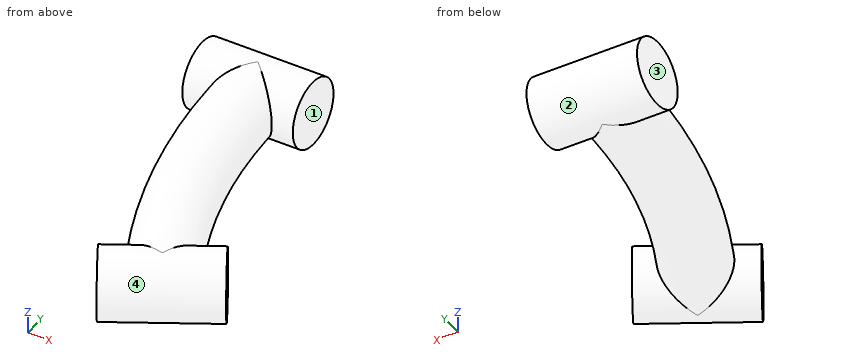
```python
from build123d import *

# Parameters (mm, degrees)
F0_R     = 3.81
F4_R     = 3.81
F5_DEPTH = 6.35
F8_R     = 3.81
F9_DEPTH = 6.35


with BuildPart() as f2:
    # F2: sweep along a path in F1
    with BuildLine(Plane.XY) as f2_path:
        ThreePointArc((0, 0), (2.5964520368, -19.7220112368), (10.2088642316, -38.1))
    # F0 (on Front) → F2 (sweep)
    with BuildSketch(Plane.XZ):
        with Locations((12.7, 0)):
            Circle(F0_R)
    sweep(path=f2_path.line)

    # F4 (on offset) → F5 (join, symmetric)
    with BuildSketch(Plane.YZ.offset(12.7)):
        Circle(F4_R)
    extrude(amount=F5_DEPTH, both=True)

    # F8 (on face) → F9 (join, symmetric)
    with BuildSketch(Plane(origin=(2.1573868597, 1.2455678842, 0), x_dir=(-0.5, 0.8660254038, 0), z_dir=(0.8660254038, 0.5, 0))):
        with Locations((-38.1, 0)):
            Circle(F8_R)
    extrude(amount=F9_DEPTH, both=True)


solid = f2.part
```
Work out the finished part from the listing and answer in its coordinate system (mm). Face numbers are marked on the shaded views. A direction names the side the tool comes from. Give positions to 0.01 mm unless a question says otherwise; leave off trailing zeros. Order: outer loops, then holes, each group sorted by start corner. A loop starts at its lowest first (then second) coordinate and runs counter-clockwise, first axis right, second up.
1. Section B-B, the plane z = -2.25 is taken. Determine the outline of the cut face in (x, y), and give its area (3 significant figures).
Result sheet:
outline: (6.35, -3.07) - (9.7, -3.07) arc R66.57 ccw to (17.07, -30.59) - (14.17, -32.26) - (17.25, -37.59) - (28.24, -31.24) - (25.17, -25.91) - (22.4, -27.51) arc R60.43 cw to (15.85, -3.07) - (19.05, -3.07) - (19.05, 3.07) - (6.35, 3.07) - close
area: 323 mm2
2. For the marked faces 1 and 2, determine the directions among +Z, -Z, +X, -X, +Y, -Y from which every point of the face is accessible in a straight line to the end or side of a thin tool.
Result sheet:
face 1: +Z, -Z, +X, +Y
face 2: none
3. Section A-A, the plane z = 1.5 is taken. Determine the outline of the cut face in (x, y).
Result sheet:
outline: (6.35, -3.5) - (9.29, -3.5) arc R67 ccw to (16.5, -30.42) - (13.96, -31.89) - (17.46, -37.96) - (28.46, -31.61) - (24.96, -25.54) - (22.58, -26.91) arc R60 cw to (16.3, -3.5) - (19.05, -3.5) - (19.05, 3.5) - (6.35, 3.5) - close
4. The mould has two halves that part along Y. Classify the marked faces 3 and 4: released by +Y, released by -Y, zero draft, split by the parting line, or undercut.
Result sheet:
face 3: zero draft
face 4: undercut
5. Straight lines are drawn through the part: L1, parallel to Z at x = 13.5, y = -11.5; L2, parallel to Y at x = 7.5, z = -0.75; L3, parallel to Y at x = 24, z = -3.25. For each, find the intervals that lie inside material, in ascending order.
Result sheet:
L1: z = -3.8 to 3.8
L2: y = -3.74 to 3.74
L3: y = -32.43 to -27.84
6. Each of these flat-tipped pins is pushed along its axis until it touches: P1, Ø1, axis at y = -16.5, z = 1.5, coming from the -X side; P2, Ø1.5, axis at y = -24.5, z = 0.5, coming from the -X side; P3, Ø1, axis at x = 24, z = -2.5, coming from the -Y side. Where does it stop, or does it pass through?
Result sheet:
P1: stops at x = 11.04
P2: stops at x = 13.24
P3: stops at y = -33.98
